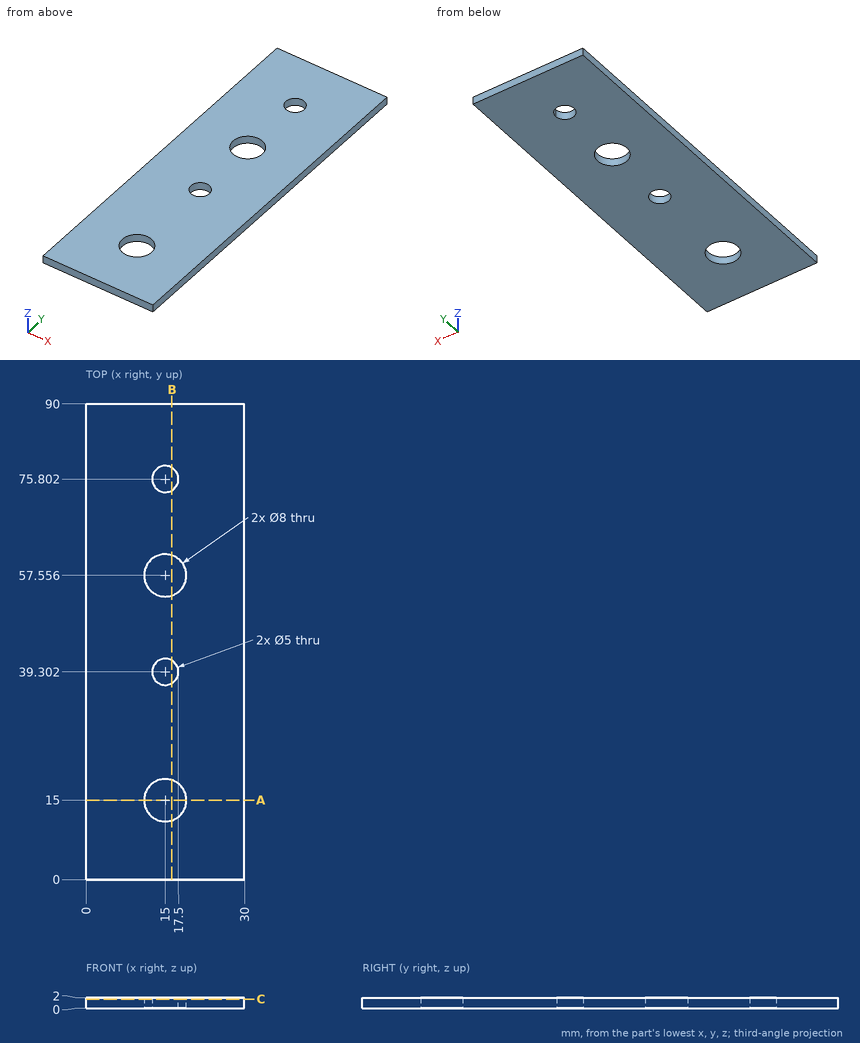
Input: dimensioned drawing with shaded views. Units: mm. Origin: part minimum x, y, z. Give positions to 0.01 mm unless a question says otherwise; leave off trailing zeros. Loops run counter-clockwise (first coordinate to the right, second up) from the corner with the lowest first, then second, coordinate; pieces in that order, holes last. Notation, with made-up numbers: (-15, -8.75) -> (37, -8.75) arc R12 ccw to (37, -3.75) -> close; hole circle Ø6 at (31.25, -31.5). An arc over 180 degrees is marked (long way). Return JSON: item names as keys, results as strings.
Item 1: Section C-C, the plane z = 1.7. Count the separate pieces of the cut face and the enclosed holes in it, plus the area to 3 significant figures.
Filled in:
{"separate pieces": "1", "enclosed holes": "4", "area": "2,560 mm^2"}
Item 2: Section B-B, the plane x = 16.25. Output: boundary loops of the cut face in (y, z).
Filled in:
{"outline": "(0, 0) -> (11.2, 0) -> (11.2, 2) -> (0, 2) -> close; (18.8, 0) -> (37.14, 0) -> (37.14, 2) -> (18.8, 2) -> close; (41.47, 0) -> (53.76, 0) -> (53.76, 2) -> (41.47, 2) -> close; (61.36, 0) -> (73.64, 0) -> (73.64, 2) -> (61.36, 2) -> close; (77.97, 0) -> (90, 0) -> (90, 2) -> (77.97, 2) -> close"}
Item 3: Pin query (flat end, axial travel): P1, Ø6.5, axis at x = 15, y = 57.56, coming from the +Z side (3 decimals); P2, Ø6, axis at x = 15, y = 75.8, coming from the +Z side. Return the tip coordinate at first contact, or that it passes through.
Filled in:
{"P1": "through", "P2": "z = 2"}
Item 4: Section A-A, the plane y = 15. Output: boundary loops of the cut face in (x, z), plus the area to 3 significant figures.
Filled in:
{"outline": "(0, 0) -> (11, 0) -> (11, 2) -> (0, 2) -> close; (19, 0) -> (30, 0) -> (30, 2) -> (19, 2) -> close", "area": "44.0 mm^2"}
Item 5: Line query: line 1 (Y direction, x = 15.5, z = 1.85) (1 decimal); line 2 (X direction, y = 16, z = 0.5); line 3 (X direction, y = 61, z = 0.8) (1 decimal). Output: solid intervals per line, ascending.
Filled in:
{"line 1": "0 to 11, 19 to 36.9, 41.8 to 53.6, 61.5 to 73.4, 78.3 to 90", "line 2": "0 to 11.13, 18.87 to 30", "line 3": "0 to 13, 17 to 30"}
